Autodesk Inventor part; units mm, degrees
ref_plane "YZ Plane" through (0, 0, 0) normal (1, 0, 0) x (0, 1, 0)
ref_plane "XZ Plane" through (0, 0, 0) normal (0, 1, 0) x (-1, 0, 0)
ref_plane "XY Plane" through (0, 0, 0) normal (0, 0, 1) x (1, 0, 0)
sketch "Sketch1" plane through (0, 0, 0) normal (0, 0, 1) x (1, 0, 0)
  line L0 (-3.9756, 0) -> (3.9756, 0)
  arc A0 (3.9756, 0) -> (1.5654, 3.6545) centre (0, 0) ccw
  line L1 (1.5654, 3.6545) -> (1.5654, 2.4102)
  line L2 (1.5654, 2.4102) -> (-1.5654, 2.4102)
  line L3 (-1.5654, 2.4102) -> (-1.5654, 3.6545)
  arc A1 (-1.5654, 3.6545) -> (-3.9756, 0) centre (0, 0) ccw
  circle A2 centre (0, 0) radius 4.075
  circle A3 centre (0, 0) radius 4.925
  line L4 (-1.5654, 3.6545) -> (-1.5654, 3.7623)
  line L5 (1.5654, 3.6545) -> (1.5654, 3.7623)
  line L6 (-4.075, 0) -> (4.2123, 0)
  line L7 (1.5654, -3.6545) -> (1.5654, -2.4102)
  line L8 (1.5654, -2.4102) -> (-1.5654, -2.4102)
  line L9 (-1.5654, -2.4102) -> (-1.5654, -3.6545)
  line L10 (-1.5654, -3.6545) -> (-1.5654, -3.7623)
  line L11 (1.5654, -3.6545) -> (1.5654, -3.7623)
  point P0 (0, 0)
  dimension "d0" = 8.15
  dimension "d1" = 9.85
extrude "Extrusion1" add sketch "Sketch1" along normal blind 15 contours L4 A2 L5 L1 L2 L3 | L10 L9 L8 L7 L11 A2 | A3
properties part number "Axel_connector"
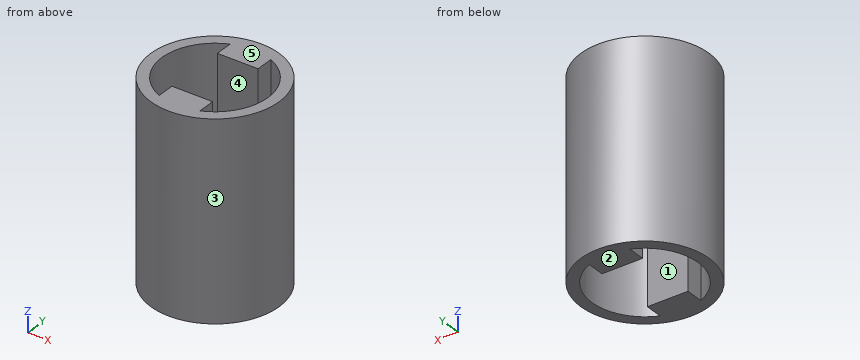
Can you work these out from the model? Positions are in its coordinate system, mm. Face numbers are marked on the shaded views. A direction names the side the tool comes from. Round coordinates to 2 decimals unless told otherwise and drop trailing zeros. Loops run counter-clockwise (first coordinate to the right, second up) from the corner with the lowest first, then second, coordinate; pieces in that order, holes last. Notation, with made-up numbers: (76, -33) -> (97, -33) arc R34 ccw to (97, -1) -> close; hole circle Ø3 at (4.5, 27.25). An arc over 180 degrees is marked (long way). One line per item, written item: value. Start each with the question number.
1. If we mould it in two halves opening along X, with no side actions, what happens to the marked faces 1, 2 and 3? For each: pulls with the +X half, pulls with the -X half, needs draft (parallel to the pull), parting line crosses it, or undercut.
2. If I drill on probe 1 along X at (y, z) = (2.75, 5); probe 2 along X at (y, z) = (3, 13); probe 3 along Y at (x, z) = (1, 9), over which ranges is the centre line in solid material (lowest first)?
3. For pin 1 (2 mm diameter, centred on y = -3, z = 3, fed in from +X); pin 2 (0.7 mm diameter, centred on y = -3, z = 7, fed in from +X); pin 3 (1.5 mm diameter, centred on x = 3.5, z = 2.5, fed in from -Y), each with a flat end and sliding along its axis, tell me the tip position at first contact or that it passes through.
4. If we section it at C-C, the plane z = 10.5: Write out the boundary of the cut face in (x, y) (3 decimals).
5. For the marked faces 4 and 5, which set-ups out of +Z, -Z, +X, -X, +Y, -Y let a thin tool reach every point of the face, with its end or its side?
6. If we section it at B-B, the plane x = 0: Write out the boundary of the cut face in (y, z) (3 decimals).
7. If we section it at A-A, the plane y = 0: Write out the boundary of the cut face in (x, z) (3 decimals), then the cut area to 3 significant figures.
Calculated:
1. face 1: undercut
1. face 2: needs draft
1. face 3: parting line crosses it
2. probe 1: x = -4.09 to -3.01, -1.57 to 1.57, 3.01 to 4.09
2. probe 2: x = -3.91 to -2.76, -1.57 to 1.57, 2.76 to 3.91
2. probe 3: y = -4.82 to -2.41, 2.41 to 4.82
3. pin 1: stops at x = 4.5
3. pin 2: stops at x = 4.15
3. pin 3: stops at y = -4.09
4. outline: circle Ø9.85 at (0, 0); hole (-1.565, -3.762) -> (-1.565, -2.41) -> (1.565, -2.41) -> (1.565, -3.762) arc R4.075 ccw to (1.565, 3.762) -> (1.565, 2.41) -> (-1.565, 2.41) -> (-1.565, 3.762) arc R4.075 ccw to start
5. face 4: +Z, -Z
5. face 5: +Z, +X, -X, +Y, -Y
6. outline: (-4.925, 0) -> (-2.41, 0) -> (-2.41, 15) -> (-4.925, 15) -> close; (2.41, 0) -> (4.925, 0) -> (4.925, 15) -> (2.41, 15) -> close
7. outline: (-4.925, 0) -> (-4.075, 0) -> (-4.075, 15) -> (-4.925, 15) -> close; (4.075, 0) -> (4.925, 0) -> (4.925, 15) -> (4.075, 15) -> close
7. area: 25.5 mm²
